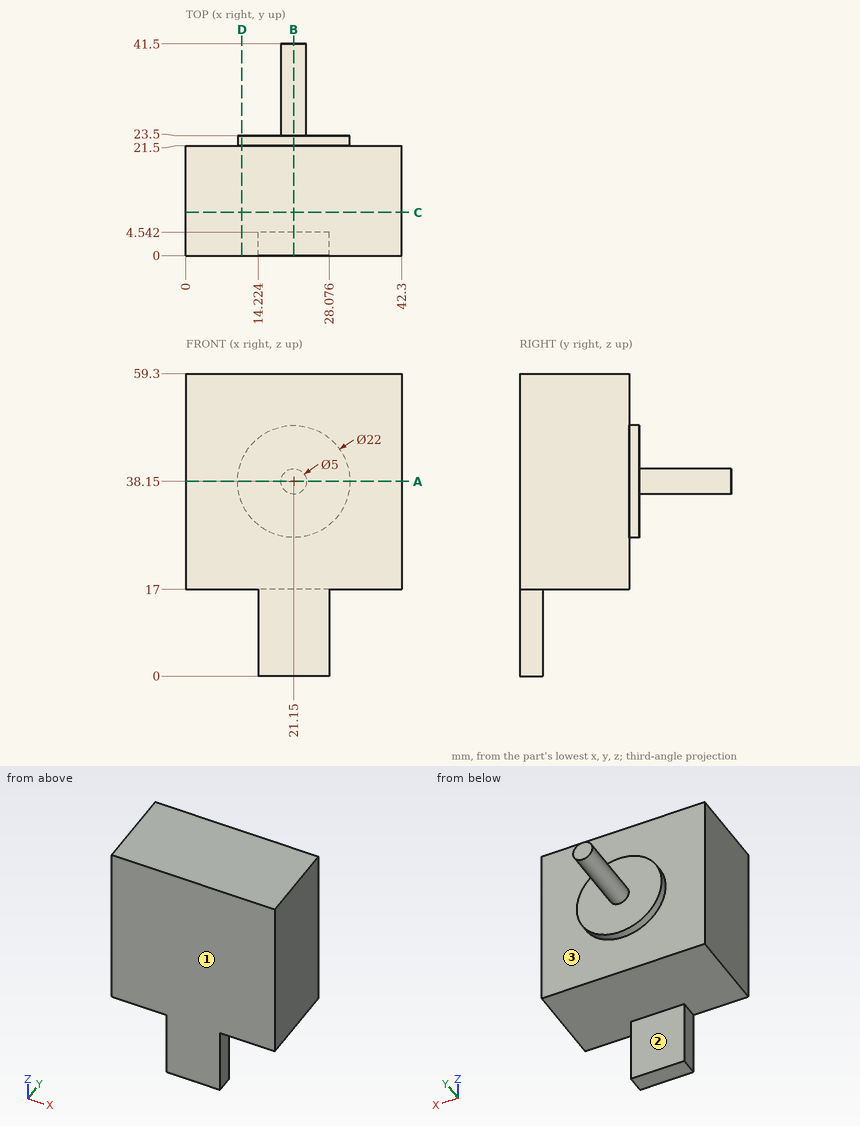
Geometry: see drawing. Coordinates: mm, zero at the bounding-box minimum. A direction names the side the tool comes from. Give positions to 0.01 mm unless a question says otherwise; leave off trailing zeros. Loops run counter-clockwise (first coordinate to the right, second up) from the corner with the lowest first, then second, coordinate; pieces in that order, holes last. Notation, with made-up numbers: (-26, -34) - (-15, -34) arc R8 cw to (-15, -25) - close; hole circle Ø7 at (21, -9). An arc over 180 degrees is marked (long way). Answer as CSV lines item,"result". Start each with the question number.
1. Reachability of the marked faces 1, 2 and 3 from +Z, -Z, +X, -X, +Y, -Y: full face, straight path, thin tool, end or side. Return the list, or none.
2. Ray query, L1, parallel to Y at x = 10, z = 51.5; L2, parallel to Y at x = 14.5, z = 36; L3, parallel to Z at x = 24, y = 20. Return the intervals inside material, ascending.
3. Section C-C, the plane y = 8.5. Return loops of the section in (x, z), plus the area to 3 significant figures.
4. Section B-B, the plane x = 21.15. Return loops of the section in (y, z), plus the area to 3 significant figures.
5. Pin query (flat end, axial travel): P1, Ø6, axis at x = 25, y = 33, coming from the +Z side; P2, Ø8, axis at x = 6.5, y = 24.5, coming from the -Z side; P3, Ø15, axis at x = 22.5, z = 10.5, coming from the +Y side; P4, Ø12, axis at x = 37.5, z = 8, coming from the -Y side. Return the tip coordinate at first contact, or that it passes through.
6. Section D-D, the plane x = 11. Return loops of the section in (y, z).
7. Section A-A, the plane z = 38.15. Return loops of the section in (x, y), plus the area to 3 significant figures.
Answers:
1,face 1,"+Z, -Z, +X, -X, -Y"
1,face 2,"-Z, +X, -X, +Y"
1,face 3,"+Y"
2,L1,"y = 0 to 21.5"
2,L2,"y = 0 to 23.5"
2,L3,"z = 17 to 59.3"
3,outline,"(0, 17) - (42.3, 17) - (42.3, 59.3) - (0, 59.3) - close"
3,area,"1,790 mm2"
4,outline,"(0, 0) - (4.54, 0) - (4.54, 17) - (21.5, 17) - (21.5, 27.15) - (23.5, 27.15) - (23.5, 35.65) - (41.5, 35.65) - (41.5, 40.65) - (23.5, 40.65) - (23.5, 49.15) - (21.5, 49.15) - (21.5, 59.3) - (0, 59.3) - close"
4,area,"1,120 mm2"
5,P1,"stops at z = 40.5"
5,P2,"stops at z = 17"
5,P3,"stops at y = 21.5"
5,P4,"passes through"
6,outline,"(0, 17) - (21.5, 17) - (21.5, 33.91) - (23.5, 33.91) - (23.5, 42.39) - (21.5, 42.39) - (21.5, 59.3) - (0, 59.3) - close"
7,outline,"(0, 0) - (42.3, 0) - (42.3, 21.5) - (32.15, 21.5) - (32.15, 23.5) - (23.65, 23.5) - (23.65, 41.5) - (18.65, 41.5) - (18.65, 23.5) - (10.15, 23.5) - (10.15, 21.5) - (0, 21.5) - close"
7,area,"1,040 mm2"
